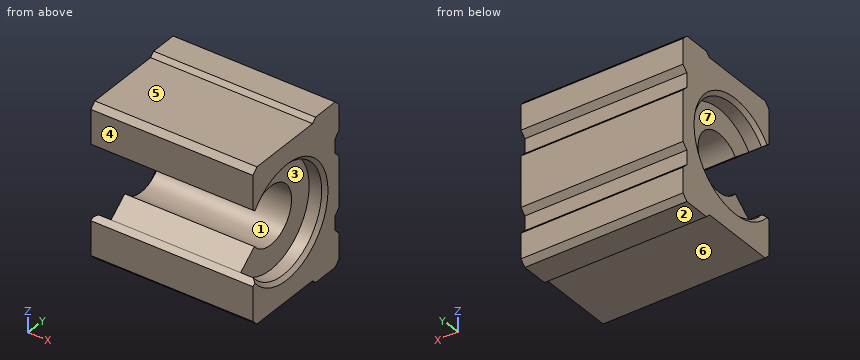
from build123d import *

# Parameters (mm, degrees)
BOSS_EXTRUDE1_DEPTH = 45
CUT_EXTRUDE1_DEPTH  = 4.5
CUT_EXTRUDE2_DEPTH  = 4.5
CHAMFER3_SIZE       = 1
CHAMFER4_SIZE       = 1
CUT_EXTRUDE3_DEPTH  = 36


with BuildPart() as part:
    # Sketch1 → Boss-Extrude1 (new body)
    with BuildSketch(Plane(origin=(0, 0, 0), x_dir=(0, 0, -1), z_dir=(1, 0, 0))):
        Polygon((-22.5, 18.5), (-21, 20), (-14, 20), (-12.5, 18.5), (-8.5, 18.5), (-7, 20), (7, 20), (8.5, 18.5), (12.5, 18.5), (14, 20), (21, 20), (22.5, 18.5), (22.5, 11), (21.36862915, 9.86862915), (21.36862915, -11.5), (19.86862915, -13), (10.408329997, -13), (9.207368844, -11.5), (-9.207368844, -11.5), (-10.408329997, -13), (-19.86862915, -13), (-21.36862915, -11.5), (-21.36862915, 9.86862915), (-22.5, 11), align=None)
    extrude(amount=BOSS_EXTRUDE1_DEPTH)

    # Sketch8 → Cut-Extrude1 (cut)
    with BuildSketch(Plane.ZY):
        with BuildLine():
            Line((-9.207368844, -11.5), (9.207368844, -11.5))
            ThreePointArc((9.207368844, -11.5), (0, 14.73179015), (-9.207368844, -11.5))
        make_face()
    extrude(amount=-CUT_EXTRUDE1_DEPTH, mode=Mode.SUBTRACT)

    # Sketch9 → Cut-Extrude2 (cut)
    with BuildSketch(Plane(origin=(45, 0, 0), x_dir=(0, 0, -1), z_dir=(1, 0, 0))):
        with BuildLine():
            Line((-9.207368844, -11.5), (9.207368844, -11.5))
            ThreePointArc((9.207368844, -11.5), (0, 14.73179015), (-9.207368844, -11.5))
        make_face()
    extrude(amount=-CUT_EXTRUDE2_DEPTH, mode=Mode.SUBTRACT)

    # Chamfer3
    chamfer3_edges = [part.edges().sort_by_distance(p)[0] for p in [
        (45, 14.73179015, 0),
    ]]
    chamfer(chamfer3_edges, length=CHAMFER3_SIZE)

    # Chamfer4
    chamfer4_edges = [part.edges().sort_by_distance(p)[0] for p in [
        (0, 14.73179015, 0),
    ]]
    chamfer(chamfer4_edges, length=CHAMFER4_SIZE)

    # Sketch10 → Cut-Extrude3 (cut)
    with BuildSketch(Plane(origin=(40.5, 0, 0), x_dir=(0, 0, -1), z_dir=(1, 0, 0))):
        with BuildLine():
            ThreePointArc((-5, -6.244997998), (0.003880032, 7.999999059), (4.99393995, -6.2498451))
            Line((4.99393995, -6.2498451), (9.207368844, -11.5))
            Line((9.207368844, -11.5), (-9.207368844, -11.5))
            Line((-9.207368844, -11.5), (-5, -6.244997998))
        make_face()
    extrude(amount=-CUT_EXTRUDE3_DEPTH, mode=Mode.SUBTRACT)


solid = part.part
For this review, take the finished solid that the model builds, in its own axes (mm). Face numbers are marked on the shaded views. A direction names the side the tool comes from. Round coordinates to 2 decimals unless told otherwise and drop trailing zeros. Loops run counter-clockwise (first coordinate to the right, second up) from the corner with the lowest first, then second, coordinate; pieces in that order, holes last. Notation, with made-up numbers: (-30.75, 78.25) - (-21.75, 78.25) arc R13 cw to (-21.75, 90.25) - close; hole circle Ø9 at (-9, 6.25). An arc over 180 degrees is marked (long way). One line per question, with ' | ' between items.
Q1. Take a section at B-B (x = 34). Give the boundary of the cut face in (y, z) (3 decimals).
Taken from the geometry:
outline: (-13, -19.869) - (-11.5, -21.369) - (9.869, -21.369) - (11, -22.5) - (18.5, -22.5) - (20, -21) - (20, -14) - (18.5, -12.5) - (18.5, -8.5) - (20, -7) - (20, 7) - (18.5, 8.5) - (18.5, 12.5) - (20, 14) - (20, 21) - (18.5, 22.5) - (11, 22.5) - (9.869, 21.369) - (-11.5, 21.369) - (-13, 19.869) - (-13, 10.408) - (-6.245, 5) arc R8 cw (long way) to (-6.25, -4.994) - (-11.5, -9.207) - (-13, -10.408) - close
Q2. For line 1 along Z through (x, y) = (42, 0); line 2 along Z through (x, y) = (9.5, -11.5); line 3 along Y through (x, z) = (13, 11), list the stretches that pass through material, from the lowest coordinate up. Write a range as [from, to].
Taken from the geometry:
line 1: z = [-21.37, -14.73], [14.73, 21.37] | line 2: z = [-21.37, -9.21], [9.21, 21.37] | line 3: y = [-13, 18.5]
Q3. Take a section at C-C (z = 0). Give the boundary of the cut face in (x, y).
Taken from the geometry:
outline: (0, 15.73) - (1, 14.73) - (4.5, 14.73) - (4.5, 8) - (40.5, 8) - (40.5, 14.73) - (44, 14.73) - (45, 15.73) - (45, 20) - (0, 20) - close
Q4. The part is to be moulded in two halves that separate along Z. For the marked faces 1, 2, 3 and 4, say which applies: released by +Z, released by -Z, zero draft, split by the parting line, or undercut.
Taken from the geometry:
face 1: undercut | face 2: released by -Z | face 3: undercut | face 4: zero draft
Q5. Tool access review of the marked faces 5, 6 and 7: name each direction out of +Z, -Z, +X, -X, +Y, -Y from which nothing blocks a thin tool from reaching the whole face with its end or side.
Taken from the geometry:
face 5: +Z, +X, -X, -Y | face 6: -Z, +X, -X, -Y | face 7: -X
Q6. Take a section at A-A (y = 0). Give the boundary of the cut face in (x, z), and give its area (3 significant figures).
Taken from the geometry:
outline: (0, -21.37) - (45, -21.37) - (45, -15.73) - (44, -14.73) - (40.5, -14.73) - (40.5, -8) - (4.5, -8) - (4.5, -14.73) - (1, -14.73) - (0, -15.73) - close; (0, 15.73) - (1, 14.73) - (4.5, 14.73) - (4.5, 8) - (40.5, 8) - (40.5, 14.73) - (44, 14.73) - (45, 15.73) - (45, 21.37) - (0, 21.37) - close | area: 1,080 mm²
Q7. For pin 1 (3 mm diameter, centred on y = 9, z = -5, fed in from +X); pin 2 (2 mm diameter, centred on x = 22.5, z = -1.5, fed in from -Y); pin 3 (1.2 mm diameter, centred on x = 27, z = -11, fed in from +Y), all flat-tipped, find the tip position at first contact; note any pin that passes through.
Taken from the geometry:
pin 1: stops at x = 40.5 | pin 2: stops at y = 7.6 | pin 3: stops at y = 18.5
